Build history of the part. All positions in model axes, mm. Give positions to 0.01 mm unless a question says otherwise; leave off trailing zeros. Write each loop counter-clockwise with the first axis right and the second up, starting at its lowest first coordinate (ties: lowest second). Pieces come first, ordered by that corner, then holes. Notation, with made-up numbers: (77.25, -26.5) -> (126.25, -26.5) arc R25 ccw to (126.25, 5.5) -> close; hole circle Ø1 at (61.5, 75.25). An arc over 180 degrees is marked (long way). Put each result on its own line as item: value. Start each with the question number.
Item 1: Slice it at A-A, the plane x = -90. List the corners of the cut face in (y, z), plus the area to 3 significant figures.
Item 2: Two-plate mould, pull along X, no slides. Class faces 1 (the flat face through (-77, 57.15, -37)), 2 (the flat face through (0, 28, -37)), 3 (the cylindrical face through (-73.65, 20.43, -7.71)), 4 (the flat face through (-77, 29, -1.27)): pulls with the +X half, pulls with the -X half, needs draft (parallel to the pull), parting line crosses it, or undercut.
Item 3: Drill centre lines: line 1 along Y through (x, z) = (-76.2, -5.25) (3 decimals); line 2 along X through (y, z) = (6, -41); line 3 along X through (y, z) = (20.32, -6). Where is each one in solid material? Low to high.
Item 4: Flat gauge pins, fed straight in: pin 1 Ø6 at (x, y) = (-76.2, 20.32) entering from +Z; pin 2 Ø0.6 at (x, z) = (-110.5, -0.5) entering from -Y. Where does each tip first touch, or does it go through?
```python
from build123d import *

# Parameters (mm, degrees)
F0_W     = 152.4
F0_H     = 57.15
F1_DEPTH = 74.3712
F2_W     = 152.4
F2_H     = 6.35
F3_DEPTH = 1.27
F5_DEPTH = 74.3722
F7_DEPTH = 1.27
F8_D     = 5.1054
F8_DEPTH = 12.7
F8_START = 1.27
F8_TIP   = 1.5338169022


with BuildPart() as f1:
    # F0 (on Top) → F1 (new body)
    with BuildSketch(Plane.XY):
        with Locations((-76.2, 28.575)):
            Rectangle(F0_W, F0_H)
    extrude(amount=-F1_DEPTH)

    # F2 (on face) → F3 (cut)
    with BuildSketch(Plane.XY):
        with Locations((-76.2, 3.175)):
            Rectangle(F2_W, F2_H)
    extrude(amount=-F3_DEPTH, mode=Mode.SUBTRACT)

    # F4 (on face) → F5 (cut, through all)
    with BuildSketch(Plane.XY):
        with BuildLine():
            Line((-79.375, 6.35), (-73.025, 6.35))
            ThreePointArc((-73.025, 6.35), (-76.2, 9.525), (-79.375, 6.35))
        make_face()
        with BuildLine():
            ThreePointArc((-79.375, 6.35), (-76.2, 3.175), (-73.025, 6.35))
            Line((-73.025, 6.35), (-79.375, 6.35))
        make_face()
    extrude(amount=-F5_DEPTH, mode=Mode.SUBTRACT)

    # F6 (on face) → F7 (cut)
    with BuildSketch(Plane.XY):
        with BuildLine():
            Line((-95.377, 6.35), (-79.375, 6.35))
            ThreePointArc((-79.375, 6.35), (-76.2, 9.525), (-73.025, 6.35))
            Line((-73.025, 6.35), (-57.023, 6.35))
            Line((-57.023, 6.35), (-57.023, 57.15))
            Line((-57.023, 57.15), (-95.377, 57.15))
            Line((-95.377, 57.15), (-95.377, 6.35))
        make_face()
    extrude(amount=-F7_DEPTH, mode=Mode.SUBTRACT)

    # F8
    # its depths count from where the whole tool has entered the part; down to there all is cleared
    with Locations(Plane.XY.offset(-F8_START)):
        with Locations((-76.2, 20.32)):
            Hole(F8_D / 2, depth=F8_DEPTH)
            with Locations((0, 0, -(F8_DEPTH + F8_TIP / 2))):  # 118° drill point
                Cone(0, F8_D / 2, F8_TIP, mode=Mode.SUBTRACT)


solid = f1.part
```
Values follow:
1. outline: (0, -74.37) -> (57.15, -74.37) -> (57.15, -1.27) -> (0, -1.27) -> close
1. area: 4,180 mm2
2. face 1: needs draft
2. face 2: pulls with the +X half
2. face 3: undercut
2. face 4: undercut
3. line 1: 0 to 3.175, 9.525 to 17.767, 22.873 to 57.15
3. line 2: -152.4 to -79.36, -73.04 to 0
3. line 3: -152.4 to -78.75, -73.65 to 0
4. pin 1: z = -1.27
4. pin 2: y = 6.35
